Model file for the job. Use its own axes, mm. Round coordinates to 2 decimals unless told otherwise and drop trailing zeros. Order: outer loops, then holes, each group sorted by start corner. A loop starts at its lowest first (then second) coordinate and runs counter-clockwise, first axis right, second up. Notation, with made-up numbers: (33, 46) - (44, 46) arc R21 ccw to (44, 82) - close; hole circle Ø10 at (82, -38.75). An arc over 180 degrees is marked (long way). Write item = value, one per line.
Autodesk Inventor part; units mm, degrees
ref_plane "YZ Plane" through (0, 0, 0) normal (1, 0, 0) x (0, 1, 0)
ref_plane "XZ Plane" through (0, 0, 0) normal (0, 1, 0) x (-1, 0, 0)
ref_plane "XY Plane" through (0, 0, 0) normal (0, 0, 1) x (1, 0, 0)
sketch "main" plane through (0, 0, 0) normal (0, 0, 1) x (1, 0, 0)
  circle A0 centre (7.297, 24.2073) radius 2.1844
  arc A1 (32.7001, 17.8573) -> (32.7001, 30.5808) centre (32.7001, 24.219) ccw
  line L0 (8.227, 9.2622) -> (15.8921, 16.9273)
  arc A2 (18.1371, 17.8573) -> (15.8921, 16.9273) centre (18.1371, 14.6823) ccw
  line L1 (32.7001, 17.8573) -> (18.1371, 17.8573)
  circle A3 centre (32.697, 24.2073) radius 2.1844
  line L2 (7.9237, 32.4766) -> (33.1809, 30.5626)
  arc A4 (7.9237, 32.4766) -> (1.1906, 29.8185) centre (7.297, 24.2073) ccw
  circle A5 centre (7.297, -26.5927) radius 2.1844
  arc A6 (-33.054, -7.4479) -> (-31.0726, -21.98) centre (-26.0405, -13.8927) ccw
  line L3 (1.381, 30.0257) -> (-33.054, -7.4479)
  arc A7 (-31.0726, -21.98) -> (7.297, -32.9427) centre (7.297, 39.6854) ccw
  line L4 (7.297, -32.9427) -> (32.697, -32.9427)
  arc A8 (32.697, -32.9427) -> (32.697, -20.2427) centre (32.697, -26.5927) ccw
  circle A9 centre (-26.0405, -13.8927) radius 2.0955
  line L5 (7.297, 7.0171) -> (7.297, -17.0677)
  arc A10 (7.297, -17.0677) -> (10.472, -20.2427) centre (10.472, -17.0677) ccw
  line L6 (10.472, -20.2427) -> (32.697, -20.2427)
  circle A11 centre (32.697, -26.5927) radius 2.1844
  arc A12 (8.227, 9.2622) -> (7.297, 7.0171) centre (10.472, 7.0171) ccw
  point P0 (10.5963, 4.2161)
  point P1 (16.822, 17.8573)
  point P2 (7.297, 8.3323)
  point P3 (1.963, 30.5573)
  point P4 (7.297, 17.8573)
  dimension "d0" = 9.525
  dimension "d1" = 9.525
  dimension "d2" = 3.175
  dimension "d3" = 4.191
  dimension "d4" = 3.175
sketch "Sketch1" plane through (0, 0, 0) normal (0, 1, 0) x (-1, 0, 0)
  circle A0 centre (-25.4, 50.8) radius 2.1844
  arc A1 (0.0031, 44.45) -> (0.0031, 57.1735) centre (0.0031, 50.8118) ccw
  line L0 (-24.4701, 35.8549) -> (-16.8049, 43.5201)
  arc A2 (-14.5599, 44.45) -> (-16.8049, 43.5201) centre (-14.5599, 41.275) ccw
  line L1 (0.0031, 44.45) -> (-14.5599, 44.45)
  circle A3 centre (0, 50.8) radius 2.1844
  line L2 (-24.7734, 59.0693) -> (0.4838, 57.1553)
  arc A4 (-24.7734, 59.0693) -> (-31.5064, 56.4112) centre (-25.4, 50.8) ccw
  circle A5 centre (-25.4, 0) radius 2.1844
  arc A6 (-65.751, 19.1448) -> (-63.7696, 4.6127) centre (-58.7375, 12.7) ccw
  line L3 (-31.316, 56.6184) -> (-65.751, 19.1448)
  arc A7 (-63.7696, 4.6127) -> (-25.4, -6.35) centre (-25.4, 66.2781) ccw
  line L4 (-25.4, -6.35) -> (0, -6.35)
  arc A8 (0, -6.35) -> (0, 6.35) centre (0, 0) ccw
  circle A9 centre (-58.7375, 12.7) radius 2.0955
  line L5 (-25.4, 33.6099) -> (-25.4, 9.525)
  arc A10 (-25.4, 9.525) -> (-22.225, 6.35) centre (-22.225, 9.525) ccw
  line L6 (-22.225, 6.35) -> (0, 6.35)
  circle A11 centre (0, 0) radius 2.1844
  arc A12 (-24.4701, 35.8549) -> (-25.4, 33.6099) centre (-22.225, 33.6099) ccw
extrude "Extrusion1" add sketch "Sketch1" along normal blind 1.5875
properties part number "gusset" material "Acetal Resin, White"
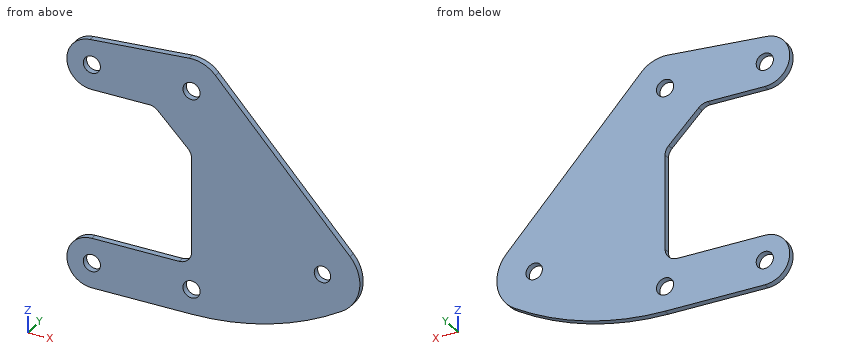
1) Flat gauge pins, fed straight in: pin 1 Ø0.5 at (y, z) = (1, 20.5) entering from -X; pin 2 Ø5 at (x, z) = (58.74, 12.7) entering from +Y; pin 3 Ø0.5 at (x, y) = (5.5, 0.5) entering from +Z. Where does each tip first touch, or does it go through?
Conclusion:
pin_1 = 25.4
pin_2 = 1.59
pin_3 = 57.63
2) Cut at D-D (x = 52). Write the cut outline in (y, z).
Conclusion:
outline = (0, -1.3) - (1.59, -1.3) - (1.59, 34.11) - (0, 34.11) - close
3) Cut at A-A (z = 12.7). Write the cut outline in (x, y).
Conclusion:
outline = (25.4, 0) - (56.64, 0) - (56.64, 1.59) - (25.4, 1.59) - close; (60.83, 0) - (68.26, 0) - (68.26, 1.59) - (60.83, 1.59) - close
4) Wall check: line 1 along Z through (x, y) = (0, 1.1); line 2 along Z through (x, y) = (4, 1.3); line 3 along X through (y, z) = (0.95, 41.5) (1 decimal). Give the ranges that are in metal, low to high.
Conclusion:
line_1 = -6.35 to -2.18, 2.18 to 6.35, 44.45 to 48.62, 52.98 to 57.19
line_2 = -6.35 to 6.35, 44.45 to 57.5
line_3 = 18.8 to 45.2
5) Cut at B-B (y = 0.7). Give the number of separate pieces and of enclosed holes in the cut face, and give its area (3 significant figures).
Conclusion:
separate_pieces = 1
enclosed_holes = 5
area = 2,540 mm^2
6) Cut at C-C (z = 52). Write the cut outline in (x, y).
Conclusion:
outline = (-6.25, 0) - (-1.83, 0) - (-1.83, 1.59) - (-6.25, 1.59) - close; (1.83, 0) - (23.57, 0) - (23.57, 1.59) - (1.83, 1.59) - close; (27.23, 0) - (35.56, 0) - (35.56, 1.59) - (27.23, 1.59) - close
